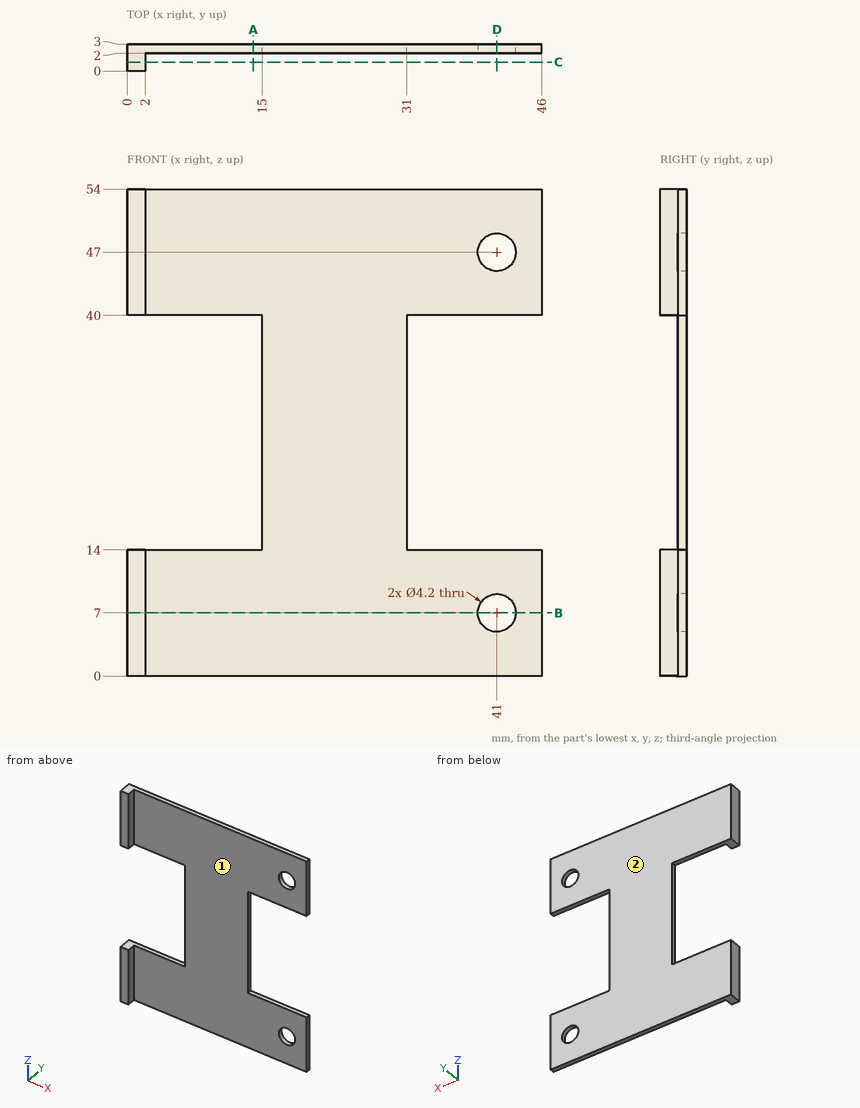
The figure shows three views and two pictorial views of one solid part (mm, origin at its lowest corner). Answer the questions. A direction names the side the tool comes from. Round coordinates to 2 decimals unless told otherwise and drop trailing zeros. Loops run counter-clockwise (first coordinate to the right, second up) from the corner with the lowest first, then second, coordinate; pieces in that order, holes last. Notation, with made-up numbers: M 2.25,72.5 L 30.25,72.5 A16 ccw 30.25,95.5 Z; hole C -25.5,20.25 d3. An arc over 180 degrees is marked long. Write each question's results on one line, items separated by ' | '. Start each with the question number.
1) Which of the six approach directions +Z, -Z, +X, -X, +Y, -Y give full straight-line access (tool end or side, diameter ignored) to the marked faces 1 and 2?
2) Find section A-A on x = 14. Write down the section's boundary in (y, z), plus the area to 3 significant figures.
3) Straight lines are drawn through the part: probe 1 along Z at (x, y) = (41, 2.6); probe 2 along Z at (x, y) = (10, 2.5); probe 3 along Z at (x, y) = (42.5, 2.4). For each, find the intervals that lie inside material, in ascending order.
4) Find section D-D on x = 41. Write down the section's boundary in (y, z).
5) Each of these flat-tipped pins is pushed along its axis until it touches: pin 1 (5 mm diameter, centred on x = 29, z = 43.5, fed in from -Y); pin 2 (1 mm diameter, centred on y = 0.5, z = 50, fed in from +X). Where does it stop, or does it pass through?
6) Find section C-C on y = 1. Write down the section's boundary in (x, z).
7) Find section B-B on z = 7. Write down the section's boundary in (x, y).
Final values:
1) face 1: +Z, -Z, +X, -Y | face 2: +Z, -Z, +X, -X, +Y
2) outline: M 2,0 L 3,0 L 3,14 L 2,14 Z; M 2,40 L 3,40 L 3,54 L 2,54 Z | area: 28.0 mm²
3) probe 1: 0 to 4.9, 9.1 to 14, 40 to 44.9, 49.1 to 54 | probe 2: 0 to 14, 40 to 54 | probe 3: 0 to 5.53, 8.47 to 14, 40 to 45.53, 48.47 to 54
4) outline: M 2,0 L 3,0 L 3,4.9 L 2,4.9 Z; M 2,9.1 L 3,9.1 L 3,14 L 2,14 Z; M 2,40 L 3,40 L 3,44.9 L 2,44.9 Z; M 2,49.1 L 3,49.1 L 3,54 L 2,54 Z
5) pin 1: y = 2 | pin 2: x = 2
6) outline: M 0,0 L 2,0 L 2,14 L 0,14 Z; M 0,40 L 2,40 L 2,54 L 0,54 Z
7) outline: M 0,0 L 2,0 L 2,2 L 38.9,2 L 38.9,3 L 0,3 Z; M 43.1,2 L 46,2 L 46,3 L 43.1,3 Z
